from build123d import *

# Parameters (mm, degrees)
P_IDAT_VYSUNUT_M1_DEPTH   = 13
ZAOBLIT1_R                = 1
SKICA6_R                  = 3.75
ODEBRAT_VYSUNUT_M4_DEPTH  = 5
SKICA7_R                  = 4.75
ODEBRAT_VYSUNUT_M5_DEPTH  = 5
P_IDAT_VYSUNUT_M2_DEPTH   = 13
SKICA9_W                  = 3.4
SKICA9_H                  = 22
ODEBRAT_VYSUNUT_M6_DEPTH  = 14
SKICA10_W                 = 14
SKICA10_H                 = 24
ODEBRAT_VYSUNUT_M7_DEPTH  = 12
SKICA11_W                 = 2.5
SKICA11_H                 = 13
P_IDAT_VYSUNUT_M3_DEPTH   = 4
SKICA12_R                 = 0.9
ODEBRAT_VYSUNUT_M8_DEPTH  = 4
SKICA13_W                 = 4
SKICA13_H                 = 11
ODEBRAT_VYSUNUT_M9_DEPTH  = 4
SKICA14_R                 = 4.5
ODEBRAT_VYSUNUT_M10_DEPTH = 4
SKICA15_W                 = 4
SKICA15_H                 = 2
P_IDAT_VYSUNUT_M4_DEPTH   = 13


with BuildPart() as part:
    # Skica1 → Přidat vysunutím1 (new body)
    with BuildSketch(Plane(origin=(0, 0, 0), x_dir=(1, 0, 0), z_dir=(0, 1, 0))):
        Polygon((0, -11), (0, 11), (-3.25, 14.25), (-30.25, 14.25), (-30.25, 16.25), (-2.421572875, 16.25), (2, 11.828427125), (2, -11.828427125), (-2.421572875, -16.25), (-30.25, -16.25), (-30.25, -14.25), (-3.25, -14.25), align=None)
    extrude(amount=P_IDAT_VYSUNUT_M1_DEPTH)

    # Zaoblit1
    zaoblit1_edges = [part.edges().sort_by_distance(p)[0] for p in [
        (-30.25, 0, -15.25),
        (-30.25, 0, 15.25),
        (-30.25, 13, 15.25),
        (-30.25, 13, -15.25),
    ]]
    fillet(zaoblit1_edges, radius=ZAOBLIT1_R)

    # Skica6 → Odebrat vysunutím4 (cut)
    with BuildSketch(Plane(origin=(0, 0, -16.25), x_dir=(-1, 0, 0), z_dir=(0, 0, -1))):
        with Locations((23.75, 6.5)):
            Circle(SKICA6_R)
    extrude(amount=-ODEBRAT_VYSUNUT_M4_DEPTH, mode=Mode.SUBTRACT)

    # Skica7 → Odebrat vysunutím5 (cut)
    with BuildSketch(Plane(origin=(0, 0, 14.25), x_dir=(-1, 0, 0), z_dir=(0, 0, -1))):
        with Locations((23.75, 6.5)):
            Circle(SKICA7_R)
    extrude(amount=-ODEBRAT_VYSUNUT_M5_DEPTH, mode=Mode.SUBTRACT)

    # Skica8 → Přidat vysunutím2 (add)
    with BuildSketch(Plane.XZ):
        Polygon((-0.343145751, 14.171572875), (20, 14.171572875), (20, -11.828427125), (2, -11.828427125), (2, 11.828427125), align=None)
    extrude(amount=-P_IDAT_VYSUNUT_M2_DEPTH)

    # Skica9 → Odebrat vysunutím6 (cut, through all)
    with BuildSketch(Plane(origin=(0, 13, 0), x_dir=(1, 0, 0), z_dir=(0, 1, 0))):
        with Locations((3.2, -1.171572875)):
            Rectangle(SKICA9_W, SKICA9_H)
    extrude(amount=-ODEBRAT_VYSUNUT_M6_DEPTH, mode=Mode.SUBTRACT)

    # Skica10 → Odebrat vysunutím7 (cut)
    with BuildSketch(Plane(origin=(0, 13, 0), x_dir=(1, 0, 0), z_dir=(0, 1, 0))):
        with Locations((13, -1.171572875)):
            Rectangle(SKICA10_W, SKICA10_H)
    extrude(amount=-ODEBRAT_VYSUNUT_M7_DEPTH, mode=Mode.SUBTRACT)

    # Skica11 → Přidat vysunutím3 (add)
    with BuildSketch(Plane(origin=(20, 0, 0), x_dir=(0, 0, -1), z_dir=(1, 0, 0))):
        with Locations((-15.421572875, 6.5)):
            Rectangle(SKICA11_W, SKICA11_H)
        with Locations((13.078427125, 6.5)):
            Rectangle(SKICA11_W, SKICA11_H)
    extrude(amount=-P_IDAT_VYSUNUT_M3_DEPTH)

    # Skica12 → Odebrat vysunutím8 (cut)
    with BuildSketch(Plane(origin=(20, 0, 0), x_dir=(0, 0, -1), z_dir=(1, 0, 0))):
        with Locations((-14.665360427, 6.555058558)):
            Circle(SKICA12_R)
        with Locations((12.322113705, 6.555061415)):
            Circle(SKICA12_R)
    extrude(amount=-ODEBRAT_VYSUNUT_M8_DEPTH, mode=Mode.SUBTRACT)

    # Skica13 → Odebrat vysunutím9 (cut)
    with BuildSketch(Plane.XY.offset(14.171572875)):
        with Locations((8.156854249, 7.5)):
            Rectangle(SKICA13_W, SKICA13_H)
    extrude(amount=-ODEBRAT_VYSUNUT_M9_DEPTH, mode=Mode.SUBTRACT)

    # Skica14 → Odebrat vysunutím10 (cut)
    with BuildSketch(Plane.ZY):
        with Locations((0, 6)):
            Circle(SKICA14_R)
    extrude(amount=-ODEBRAT_VYSUNUT_M10_DEPTH, mode=Mode.SUBTRACT)

    # Skica15 → Přidat vysunutím4 (add)
    with BuildSketch(Plane(origin=(0, 13, 0), x_dir=(1, 0, 0), z_dir=(0, 1, 0))):
        with Locations((-15, 13.25)):
            Rectangle(SKICA15_W, SKICA15_H)
    extrude(amount=-P_IDAT_VYSUNUT_M4_DEPTH)


solid = part.part
Input: part model. Units: mm. Frame: model coordinates. A direction names the side the tool comes from. Give positions to 0.01 mm unless a question says otherwise; leave off trailing zeros. Write each loop counter-clockwise with the first axis right and the second up, starting at its lowest first coordinate (ties: lowest second). Pieces come first, ordered by that corner, then holes. Notation, with made-up numbers: M 43.25,-12.75 L 99.25,-12.75 A5 ccw 99.25,-5.75 Z; hole C 56.25,81.25 d9. An arc over 180 degrees is marked long. Use one line per item in the form item = value.
1. Reachability of faces 1 (the face through (10.157, 7, 14)), 2 (the face through (-1.37, 6.41, 15.2)), 3 (the face through (-2, 6, 13)), 4 (the face through (-0.24, 6.41, -14.07)), 5 (the face through (13, 7, -10.828)) from +Z, -Z, +X, -X, +Y, -Y: full face, straight path, thin tool, end or side. Return the list, or none.
Outcome:
face_1 = +Z, +Y
face_2 = +Z, +Y, -Y
face_3 = -X, +Y, -Y
face_4 = -Z, +Y, -Y
face_5 = +X, +Y
2. Ray query, L1, parallel to X at y = 10.5, z = 7; L2, parallel to X at y = 3, z = 15; L3, parallel to Y at x = 0.6, z = 0. Return the intervals inside material, ascending.
Outcome:
L1 = 0 to 1.5, 4.9 to 6
L2 = -30.25 to -26.96, -20.54 to -1.17, 16 to 20
L3 = 0 to 1.5, 10.5 to 13
3. Cut plane C-C on x = -23.75. Return loops of the section in (y, z), and give its area (3 significant figures).
Outcome:
outline = M 0,-16.25 L 2.75,-16.25 L 2.75,-14.25 L 0,-14.25 Z; M 0,14.25 L 1.75,14.25 L 1.75,16.25 L 0,16.25 Z; M 10.25,-16.25 L 13,-16.25 L 13,-14.25 L 10.25,-14.25 Z; M 11.25,14.25 L 13,14.25 L 13,16.25 L 11.25,16.25 Z
area = 18.0 mm²
4. Cut plane A-A on x = -15.5. Return loops of the section in (y, z), and give its area (3 significant figures).
Outcome:
outline = M 0,-16.25 L 13,-16.25 L 13,-12.25 L 0,-12.25 Z; M 0,14.25 L 13,14.25 L 13,16.25 L 0,16.25 Z
area = 78.0 mm²
5. First-contact query: P1, Ø3.5, axis at x = 4, y = 4, coming from the +Z side; P2, Ø7, axis at y = 6, z = 0, coming from the -X side; P3, Ø1, axis at y = 11.5, z = -1, coming from the +X side. Flat tips, straight axial feed; report the tip coordinate or a pass-through.
Outcome:
P1 = 14.17
P2 = 4.9
P3 = 6
6. Mould query, pull axis Y, two halves, no side actions, for faces 6 (the face through (-25.48, 3.173, -15.264)), 7 (the face through (0.74, 1.61, -0.98)), 8 (the face through (-29.965, 0.301, -15.264)), 9 (the face through (0, 11, 0)). Classes: released by +Y, released by -Y, zero draft, split by the parting line, or undercut.
Outcome:
face_6 = undercut
face_7 = undercut
face_8 = released by -Y
face_9 = zero draft
7. Cut plane B-B on z = 0. Return loops of the section in (x, y), and give its area (3 significant figures).
Outcome:
outline = M 0,0 L 1.5,0 L 1.5,1.5 L 0,1.5 Z; M 0,10.5 L 1.5,10.5 L 1.5,13 L 0,13 Z; M 4.9,0 L 20,0 L 20,1 L 6,1 L 6,13 L 4.9,13 Z
area = 34.3 mm²
8. Cut plane D-D on z = 7. Return loops of the section in (x, y), and give its area (3 significant figures).
Outcome:
outline = M 0,0 L 1.5,0 L 1.5,13 L 0,13 Z; M 4.9,0 L 20,0 L 20,1 L 6,1 L 6,13 L 4.9,13 Z
area = 47.8 mm²
